```python
from build123d import *

# Parameters (mm, degrees)
SKETCH1_W           = 115.8875
SKETCH1_H           = 114.3
SKETCH1_W_2         = 33.3375
SKETCH1_H_2         = 66.675
BOSS_EXTRUDE1_DEPTH = 6.35
SKETCH2_W           = 112.7125
SKETCH2_H           = 111.125
CUT_EXTRUDE1_DEPTH  = 4.7625
FILLET2_R           = 6.35


with BuildPart() as part:
    # Sketch1 → Boss-Extrude1 (new body)
    with BuildSketch(Plane.XY):
        Rectangle(SKETCH1_W, SKETCH1_H)
        with Locations((-23.820216951, 0)):
            Rectangle(SKETCH1_W_2, SKETCH1_H_2, mode=Mode.SUBTRACT)
        with Locations((23.8125, 0)):
            Rectangle(SKETCH1_W_2, SKETCH1_H_2, mode=Mode.SUBTRACT)
    extrude(amount=BOSS_EXTRUDE1_DEPTH)

    # Sketch2 → Cut-Extrude1 (cut)
    with BuildSketch(Plane(origin=(0, 0, 0), x_dir=(-1, 0, 0), z_dir=(0, 0, -1))):
        Rectangle(SKETCH2_W, SKETCH2_H)
    extrude(amount=-CUT_EXTRUDE1_DEPTH, mode=Mode.SUBTRACT)

    # Fillet2
    # the kernel refuses this fillet: 6.35 mm, written as the material it adds along each edge
    with BuildSketch(Plane(origin=(56.35625, -55.5625, 4.7625), x_dir=(0, 0, -1), z_dir=(-1, 0, 0)), Plane(origin=(-56.35625, 55.5625, 4.7625), x_dir=(0, 0, -1), z_dir=(1, 0, 0))) as fillet2_piece_1:
        with BuildLine():
            CenterArc((6.35, -6.148361062), FILLET2_R, 104.477512186, 75.522487814)
            Line((0, -6.148361062), (0, 0))
            Line((0, 0), (4.7625, 0))
        make_face()
    extrude(amount=112.7125)
    with BuildSketch(Plane(origin=(-56.35625, -55.5625, 4.7625), x_dir=(0, 0, -1), z_dir=(0, 1, 0)), Plane(origin=(56.35625, 55.5625, 4.7625), x_dir=(0, 0, -1), z_dir=(0, -1, 0))) as fillet2_piece_2:
        with BuildLine():
            CenterArc((6.35, -6.148361062), FILLET2_R, 104.477512186, 75.522487814)
            Line((0, -6.148361062), (0, 0))
            Line((0, 0), (4.7625, 0))
        make_face()
    extrude(amount=111.125)
    # the kernel refuses this fillet: 6.35 mm, written as the material it takes off along each edge
    with BuildSketch(Plane(origin=(-73.81875, 57.15, 6.35), x_dir=(0, 0, -1), z_dir=(1, 0, 0))) as fillet2_2_piece_1:
        with BuildLine():
            CenterArc((FILLET2_R, -FILLET2_R), FILLET2_R, 90, 90)
            Line((0, -FILLET2_R), (0, 0))
            Line((0, 0), (FILLET2_R, 0))
        make_face()
    extrude(amount=147.6375, mode=Mode.SUBTRACT)
    with BuildSketch(Plane(origin=(-57.94375, -73.025, 6.35), x_dir=(0, 0, -1), z_dir=(0, 1, 0)), Plane(origin=(57.94375, 73.025, 6.35), x_dir=(0, 0, -1), z_dir=(0, -1, 0))) as fillet2_2_piece_2:
        with BuildLine():
            CenterArc((FILLET2_R, -FILLET2_R), FILLET2_R, 90, 90)
            Line((0, -FILLET2_R), (0, 0))
            Line((0, 0), (FILLET2_R, 0))
        make_face()
    extrude(amount=146.05, mode=Mode.SUBTRACT)
    with BuildSketch(Plane(origin=(73.81875, -57.15, 6.35), x_dir=(0, 1, 0), z_dir=(-1, 0, 0))) as fillet2_2_piece_3:
        with BuildLine():
            CenterArc((FILLET2_R, FILLET2_R), FILLET2_R, 180, 90)
            Line((0, FILLET2_R), (0, 0))
            Line((0, 0), (FILLET2_R, 0))
        make_face()
    extrude(amount=147.6375, mode=Mode.SUBTRACT)


solid = part.part
```
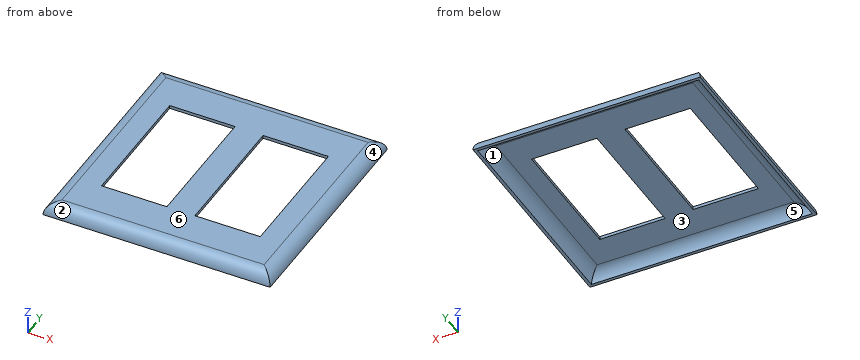
CAD build for the part. Positions are in the model's coordinates, mm. Face numbers are marked on the shaded views. A direction names the side the tool comes from. Round coordinates to 2 decimals unless told otherwise and drop trailing zeros. Write each loop counter-clockwise with the first axis right and the second up, starting at its lowest first coordinate (ties: lowest second). Pieces come first, ordered by that corner, then holes. Notation, with made-up numbers: M 48,88.5 L 92,88.5 A31 cw 92,114.5 Z; hole C 73,23.25 d6. An arc over 180 degrees is marked long. One line per question, with ' | ' between items.
1. Cut at A-A on x = -28. Write the cut outline in (y, z), and give its area (3 significant figures).
Working result:
outline: M -57.15,0 L -55.56,0 A6.35 cw -49.41,4.76 L -33.34,4.76 L -33.34,6.35 L -50.8,6.35 A6.35 ccw Z; M 33.34,4.76 L 49.41,4.76 A6.35 cw 55.56,0 L 57.15,0 A6.35 ccw 50.8,6.35 L 33.34,6.35 Z | area: 88.6 mm2
2. Pin check, flat tips, straight feed: pin 1 Ø8 at (x, y) = (13.5, 10) entering from -Z; pin 2 Ø1.7 at (x, z) = (-26, 5.5) entering from +Y; pin 3 Ø1.3 at (y, z) = (15.5, 5) entering from -X; pin 4 Ø0.5 at (x, z) = (23, 5.5) entering from +Y. Stop position of each tip, or through.
Working result:
pin 1: through | pin 2: y = 55.12 | pin 3: x = -56.22 | pin 4: y = 54.37
3. Cut at B-B on y = 0.5. Write the cut outline in (x, z), and give its area (3 significant figures).
Working result:
outline: M -57.94,0 L -56.36,0 A6.35 cw -50.21,4.76 L -40.49,4.76 L -40.49,6.35 L -51.59,6.35 A6.35 ccw Z; M -7.15,4.76 L 7.14,4.76 L 7.14,6.35 L -7.15,6.35 Z; M 40.48,4.76 L 50.21,4.76 A6.35 cw 56.36,0 L 57.94,0 A6.35 ccw 51.59,6.35 L 40.48,6.35 Z | area: 91.1 mm2
4. Probe L1, parallel to Z at x = 12.5, y = -45; L2, parallel to Y at x = 31, z = 5.25; L3, parallel to X at y = 46.5, z = 3.5. List the from-to ranges inside material, lowest first. Write a range as from..to.
Working result:
L1: 4.76..6.35 | L2: -54.37..-33.34, 33.34..54.37 | L3: -56.89..-54.01, 54.01..56.89
5. Mould opens along X. For the marked faces 1, 2, 3 and 4 say: pulls with the +X half, pulls with the -X half, needs draft (parallel to the pull), parting line crosses it, or undercut.
Working result:
face 1: undercut | face 2: needs draft | face 3: undercut | face 4: pulls with the +X half
6. Cut at C-C on z = 1.75. Write the cut outline in (x, y).
Working result:
outline: M -57.7,-56.9 L 57.7,-56.9 L 57.7,56.9 L -57.7,56.9 Z; hole M -55.61,-54.82 L 55.61,-54.82 L 55.61,54.82 L -55.61,54.82 Z
7. Cut at D-D on y = 42. Write the cut outline in (x, z).
Working result:
outline: M -57.94,0 L -56.36,0 A6.35 cw -50.21,4.76 L 50.21,4.76 A6.35 cw 56.36,0 L 57.94,0 A6.35 ccw 51.59,6.35 L -51.59,6.35 A6.35 ccw Z
8. Which spindle directions (+Z, -Z, +X, -X, +Y, -Y) get a long thin tool onto all of the face, cutting with end or side? Do the marked faces 5 and 6. Say none if no direction does.
Working result:
face 5: -Z | face 6: +Z, +X, -X, +Y, -Y
